from build123d import *

# Parameters (mm, degrees)
BOSS_EXTRUDE1_DEPTH     = 4
BOSS_EXTRUDE2_DEPTH     = 4.5
CUT_EXTRUDE1_DEPTH      = 99.435547891
CUT_EXTRUDE1_DEPTH_BACK = 99.435547891
CUT_EXTRUDE2_START      = -4.5
CUT_EXTRUDE2_DEPTH      = 4.5
CUT_EXTRUDE3_DEPTH      = 95.023100537
CUT_EXTRUDE3_DEPTH_BACK = 95.023100537
CUT_EXTRUDE4_DEPTH      = 94.998158329
CUT_EXTRUDE4_DEPTH_BACK = 94.998158329
SKETCH6_W               = 15.7
SKETCH6_H               = 4.5
FILLET1_R               = 3
BOSS_EXTRUDE3_DEPTH     = 0.7
CUT_EXTRUDE5_DEPTH      = 94.967813764
CUT_EXTRUDE5_DEPTH_BACK = 94.967813764
SKETCH8_R               = 3.15


# Read off the part's stored shape, not the designer's step: Cut-Extrude2
with BuildPart() as part:
    # Sketch1 → Boss-Extrude1 (new body)
    with BuildSketch(Plane(origin=(0, 0, 0), x_dir=(1, 0, 0), z_dir=(0, 1, 0))):
        Polygon((-15.85, -91.997703776), (15.85, -91.997703776), (17.15, 91.997703776), (-17.15, 91.997703776), align=None)
    extrude(amount=BOSS_EXTRUDE1_DEPTH)

    # Sketch2 → Boss-Extrude2 (add)
    with BuildSketch(Plane(origin=(0, 4, 0), x_dir=(1, 0, 0), z_dir=(0, 1, 0))):
        Polygon((-8.349812803, -91.997703776), (8.349812803, -91.997703776), (9.649812803, 91.997703776), (-9.649812803, 91.997703776), align=None)
    extrude(amount=BOSS_EXTRUDE2_DEPTH)

    # Sketch3 → Cut-Extrude1 (cut, two sides: drawn at the far end of the back side and taken through both)
    with BuildSketch(Plane(origin=(16.499176365, 0, 0.116573177), x_dir=(0.007065217391304343, 0, -0.9999750410401319), z_dir=(0.999975041040132, 0, 0.0070652173913043435)).offset(-CUT_EXTRUDE1_DEPTH_BACK)):
        Polygon((92.116576087, 0), (81.116576087, 8.5), (92.116576087, 8.5), align=None)
    extrude(amount=CUT_EXTRUDE1_DEPTH + CUT_EXTRUDE1_DEPTH_BACK, mode=Mode.SUBTRACT)

    # Cut-Extrude2 outline → Cut-Extrude2 (cut)
    with BuildSketch(Plane(origin=(0, 8.5, 0), x_dir=(1, 0, 0), z_dir=(0, 1, 0)).offset(CUT_EXTRUDE2_START)):
        with BuildLine():
            ThreePointArc((8.440819946, -79.117014334), (0.10345841, -87.440771539), (-8.439329356, -79.327984806))
            Line((-8.439329356, -79.327984806), (-8.349812803, -91.997703776))
            Line((-8.349812803, -91.997703776), (8.349812803, -91.997703776))
            Line((8.349812803, -91.997703776), (8.440819946, -79.117014334))
        make_face()
    extrude(amount=CUT_EXTRUDE2_DEPTH, mode=Mode.SUBTRACT)

    # Sketch5 → Cut-Extrude3 (cut, two sides: drawn at the far end of the back side and taken through both)
    with BuildSketch(Plane(origin=(0, 0, 0.056470136), x_dir=(0, 0, -1), z_dir=(1, 0, 0)).offset(-CUT_EXTRUDE3_DEPTH_BACK)):
        Polygon((-91.941233639, 0), (-90.441233639, 4), (-91.941233639, 4), align=None)
    extrude(amount=CUT_EXTRUDE3_DEPTH + CUT_EXTRUDE3_DEPTH_BACK, mode=Mode.SUBTRACT)

    # Sketch6 → Cut-Extrude4 (cut, two sides: drawn at the far end of the back side and taken through both)
    with BuildSketch(Plane(origin=(0, 0, 0.030994299), x_dir=(0, 0, -1), z_dir=(1, 0, 0)).offset(-CUT_EXTRUDE4_DEPTH_BACK)):
        with Locations((-42.060436633, 6.25)):
            Rectangle(SKETCH6_W, SKETCH6_H)
    extrude(amount=CUT_EXTRUDE4_DEPTH + CUT_EXTRUDE4_DEPTH_BACK, mode=Mode.SUBTRACT)

    # Fillet1
    fillet1_edges = [part.edges().sort_by_distance(p)[0] for p in [
        (13.363520706, 4, -86.847856952),
        (-13.364854981, 4, -87.03670345),
    ]]
    fillet(fillet1_edges, radius=FILLET1_R)

    # Fillet3
    # an asymmetric fillet: 5, 3 mm, written as the material it takes off along each edge
    with BuildSketch(Plane(origin=(-15.891485902, 15.657877718, 86.125999632), x_dir=(-0.006615348832314233, -0.3511311249673921, -0.9363029265355098), z_dir=(0.002480817730747878, -0.9363262962659619, 0.3511223610997357))) as fillet3_piece_1:
        with BuildLine():
            Bezier((2.966988077, 0), (0, 0), (-0.032946278, 4.980153892), weights=[1, 0.709441812, 1])
            Line((-0.032946278, 4.980153892), (0, 0))
            Line((0, 0), (2.966988077, 0))
        make_face()
    extrude(amount=29.173329366, mode=Mode.SUBTRACT)
    with BuildSketch(Plane(origin=(15.819112189, -11.657877718, 96.36940792), x_dir=(-0.9999969227669587, 0.002322862025529483, -0.0008710732595747153), z_dir=(0.002480817730747878, 0.9363262962659619, -0.3511223610997357))) as fillet3_piece_2:
        with BuildLine():
            Bezier((4.98026287, 0), (0, 0), (-0.019627722, -2.966923154), weights=[1, 0.709441812, 1])
            Line((-0.019627722, -2.966923154), (0, 0))
            Line((0, 0), (4.98026287, 0))
        make_face()
    extrude(amount=29.173329366, mode=Mode.SUBTRACT)

    # Sketch7 → Boss-Extrude3 (add)
    with BuildSketch(Plane(origin=(0, 4, 0), x_dir=(1, 0, 0), z_dir=(0, 1, 0))):
        Polygon((-8.64695693, -49.941430932), (-8.757883612, -34.241430932), (8.757883612, -34.241430932), (8.64695693, -49.941430932), align=None)
    extrude(amount=BOSS_EXTRUDE3_DEPTH)

    # Sketch8 → Cut-Extrude5 (cut, two sides: drawn at the far end of the back side and taken through both)
    with BuildSketch(Plane(origin=(0, 8.5, 0), x_dir=(1, 0, 0), z_dir=(0, 1, 0)).offset(-CUT_EXTRUDE5_DEPTH_BACK)):
        with Locations(Location((0, -58.002296224, 0), (0, 0, 270))):
            Circle(SKETCH8_R)
        with Locations(Location((0, 56.997703776, 0), (0, 0, 270))):
            Circle(SKETCH8_R)
        with Locations(Location((0, 41.997703776, 0), (0, 0, 270))):
            Circle(SKETCH8_R)
    extrude(amount=CUT_EXTRUDE5_DEPTH + CUT_EXTRUDE5_DEPTH_BACK, mode=Mode.SUBTRACT)


solid = part.part
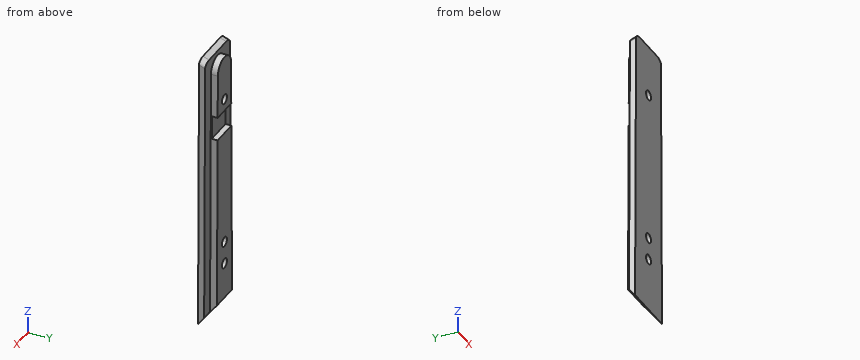
Input: part model. Units: mm. Frame: model coordinates. Give positions to 0.01 mm unless a question says otherwise; leave off trailing zeros. Write each loop counter-clockwise with the first axis right and the second up, starting at its lowest first coordinate (ties: lowest second). Pieces come first, ordered by that corner, then holes. Notation, with made-up numbers: (18, -15.5) -> (77, -15.5) arc R23 cw to (77, 13.5) -> close; hole circle Ø6 at (71, 0.25). An arc over 180 degrees is marked (long way). Use one line per item in the form item = value. Start each with the question number.
1) Section query B-B on z = -23. Return the cut outline in (x, y).
2) Pin query (flat end, axial travel): pin 1 (3 mm diameter, centred on x = 0.5, y = 7.5, fed in from +Z); pin 2 (4 mm diameter, centred on x = 4, y = 6.5, fed in from -Z); pin 3 (4 mm diameter, centred on x = 0, z = -57, fed in from -Y); pin 4 (4 mm diameter, centred on x = -10, y = 5.5, fed in from +Z). Return the tip coordinate at first contact, or that it passes through.
3) Section query A-A on x = 0. Return the cut outline in (y, z), then the cut area to 3 significant figures.
4) Ray query, probe 1 along Z at (x, y) = (0, 4.75); probe 2 along Z at (x, y) = (0, 5.75); probe 3 along Z at (x, y) = (2, 4.5). Return the intervals inside material, ascending. Write a range as from..to.
Outcome:
q1.outline = (-16.66, 0) -> (16.66, 0) -> (16.66, 4) -> (9.16, 4) -> (9.16, 8.5) -> (-9.16, 8.5) -> (-9.16, 4) -> (-16.66, 4) -> close
q2.pin_1 = 87.44
q2.pin_2 = -86.27
q2.pin_3 = through
q2.pin_4 = 90.69
q3.outline = (0, -92) -> (0.09, -92) -> (8.5, -81.12) -> (8.5, -60.15) -> (0, -60.15) -> close; (0, -53.85) -> (8.5, -53.85) -> (8.5, -45.15) -> (0, -45.15) -> close; (0, -38.85) -> (8.5, -38.85) -> (8.5, 34.24) -> (4.7, 34.24) -> (4.7, 49.94) -> (8.5, 49.94) -> (8.5, 54.85) -> (0, 54.85) -> close; (0, 61.15) -> (8.5, 61.15) -> (8.5, 87.44) -> (4, 87.44) -> (4, 90.5) -> (0, 92) -> close
q3.area = 1,270 mm^2
q4.probe_1 = -85.97..-60.15, -53.85..-45.15, -38.85..34.24, 49.94..54.85, 61.15..87.44
q4.probe_2 = -84.68..-60.15, -53.85..-45.15, -38.85..34.24, 49.94..54.85, 61.15..87.44
q4.probe_3 = -86.28..-59.43, -54.56..-44.43, -39.56..55.57, 60.44..87.2
